Autodesk Fusion 360 part; units mm, degrees
sketch "Sketch1" plane through (0, 0, 0) normal (0, 0, 1) x (1, 0, 0) in component "Spectroscope Feet"
  circle A0 centre (96.1288, 55.5) radius 6
  circle A1 centre (-96.1288, 55.5) radius 6
  circle A2 centre (0, -111) radius 6
  circle A3 centre (0, -111) radius 7.5
  circle A4 centre (-96.1288, 55.5) radius 7.5
  circle A5 centre (96.1288, 55.5) radius 7.5
  circle A6 centre (0, 0) radius 10
  line L0 (92.3788, 61.9952) -> (1.9782, 9.8024)
  line L1 (99.8788, 49.0048) -> (9.4782, -3.188)
  line L2 (-99.8788, 49.0048) -> (-9.4782, -3.188)
  line L3 (-92.3788, 61.9952) -> (-1.9782, 9.8024)
  line L4 (-7.5, -111) -> (-7.5, -6.6144)
  line L5 (7.5, -111) -> (7.5, -6.6144)
  circle A7 centre (0, 0) radius 5
  dimension "d4" = 12
  dimension "d5" = 12
  dimension "d6" = 12
  dimension "d7" = 15
  dimension "d8" = 15
  dimension "d9" = 15
  dimension "d10" = 20
  dimension "d11" = 10
extrude "Extrude1" add sketch "Sketch1" along normal blind 5 in component "Spectroscope Feet"
component "Spectroscope Feet" placed x (1, 0, 0) y (0, 1, 0) z (0, 0, 1) at (0, 0, 0)
Here's how the part is built. I have some questions about the finished solid (model axes, mm). A direction names the side the tool comes from. Coordinates: 2 decimals unless noted, no trailing zeros. Write each loop counter-clockwise with the first axis right and the second up, starting at its lowest first coordinate (ties: lowest second). Pieces come first, ordered by that corner, then holes. Notation, with made-up numbers: (86, -2.75) - (119, -2.75) arc R16 ccw to (119, 1.25) - close; hole circle Ø2 at (47.25, -32). An arc over 180 degrees is marked (long way). Use one line per item in the form item = value.
1) Suppose I cut it at B-B, the plane y = 0. Write out the boundary of the cut face in (x, z).
Solved:
outline = (-15, 0) - (-5, 0) - (-5, 5) - (-15, 5) - close; (5, 0) - (15, 0) - (15, 5) - (5, 5) - close
2) Thinking about a two-plate mould opening in Y: for faces 1 (the flat face through (-47.811, 36.264, 2.465)), 2 (the flat face through (55.311, 23.274, 2.465)), 3 (the cylindrical face through (-0.78, -116.95, 2.46)), which applies, released by +Y, released by -Y, zero draft, split by the parting line, or undercut?
Solved:
face_1 = released by +Y
face_2 = released by -Y
face_3 = undercut
3) I need wall thicknesses on line 1 (X direction, y = -38, z = 1.05); line 2 (X direction, y = 42, z = 2.9); line 3 (X direction, y = 47, z = 3.4). Which ranges of each line are inside material? Lowest first, please.
Solved:
line_1 = -7.5 to 7.5
line_2 = -87.75 to -57.75, 57.75 to 87.75
line_3 = -96.41 to -66.41, 66.41 to 96.41
4) Suppose I cut it at C-C, the plane y = 55.5. Write out the boundary of the cut face in (x, z), plus the area to 3 significant figures.
Solved:
outline = (-103.63, 0) - (-102.13, 0) - (-102.13, 5) - (-103.63, 5) - close; (-90.13, 0) - (-81.13, 0) - (-81.13, 5) - (-90.13, 5) - close; (81.13, 0) - (90.13, 0) - (90.13, 5) - (81.13, 5) - close; (102.13, 0) - (103.63, 0) - (103.63, 5) - (102.13, 5) - close
area = 105 mm2
5) On a 3-axis mill with a long thin cutter (end or side, diameter ignored), from which of +Z, -Z, +X, -X, +Y, -Y can I reach the whole of each face in a straight line? I mean faces 4 (the flat face through (47.811, 36.264, 2.465)), 5 (the cylindrical face through (102.54, 59.39, 2.46)), 6 (the flat face through (-7.5, -60, 2)), 7 (the cylindrical face through (0.16, -118.5, 2.46)), 8 (the flat face through (7.5, -60, 2)). Say none if no direction works.
Solved:
face_4 = +Z, -Z, +Y
face_5 = +Z, -Z
face_6 = +Z, -Z, -X, -Y
face_7 = +Z, -Z, -Y
face_8 = +Z, -Z, +X, -Y
6) I'm going to push flat-ended pins straight in: P1, Ø2, axis at x = 7, z = 1, coming from the +Y side; P2, Ø1, axis at y = -79, z = 4, coming from the +X side. Where does each tip first touch, or does it pass through?
Solved:
P1 = 13.28
P2 = 7.5
7) Suppose I cut it at D-D, the plane y = -22.5. Write out the boundary of the cut face in (x, z), plus the area to 3 significant figures.
Solved:
outline = (-7.5, 0) - (7.5, 0) - (7.5, 5) - (-7.5, 5) - close
area = 75.0 mm2
8) Suppose I cut it at A-A, the plane z = 3.9. Write out the boundary of the cut face in (x, y).
Solved:
outline = (-99.88, 49) - (-9.48, -3.19) arc R10 ccw to (-7.5, -6.61) - (-7.5, -111) arc R7.5 ccw to (7.5, -111) - (7.5, -6.61) arc R10 ccw to (9.48, -3.19) - (99.88, 49) arc R7.5 ccw to (92.38, 62) - (1.98, 9.8) arc R10 ccw to (-1.98, 9.8) - (-92.38, 62) arc R7.5 ccw to start; hole circle Ø12 at (-96.13, 55.5); hole circle Ø12 at (0, -111); hole circle Ø10 at (0, 0); hole circle Ø12 at (96.13, 55.5)
